Geometry check sheet. Reference: drawing and pictorial views, mm from the part's lowest x, y, z. Round coordinates to 2 decimals unless told otherwise and drop trailing zeros. Write each loop counter-clockwise with the first axis right and the second up, starting at its lowest first coordinate (ties: lowest second). Pieces come first, ordered by that corner, then holes. Notation, with made-up numbers: (-6, 25.25) - (22, 25.25) arc R34 cw to (22, 59.25) - close; hole circle Ø1 at (-17, 19). An arc over 180 degrees is marked (long way). Return JSON: item names as keys, results as strings.
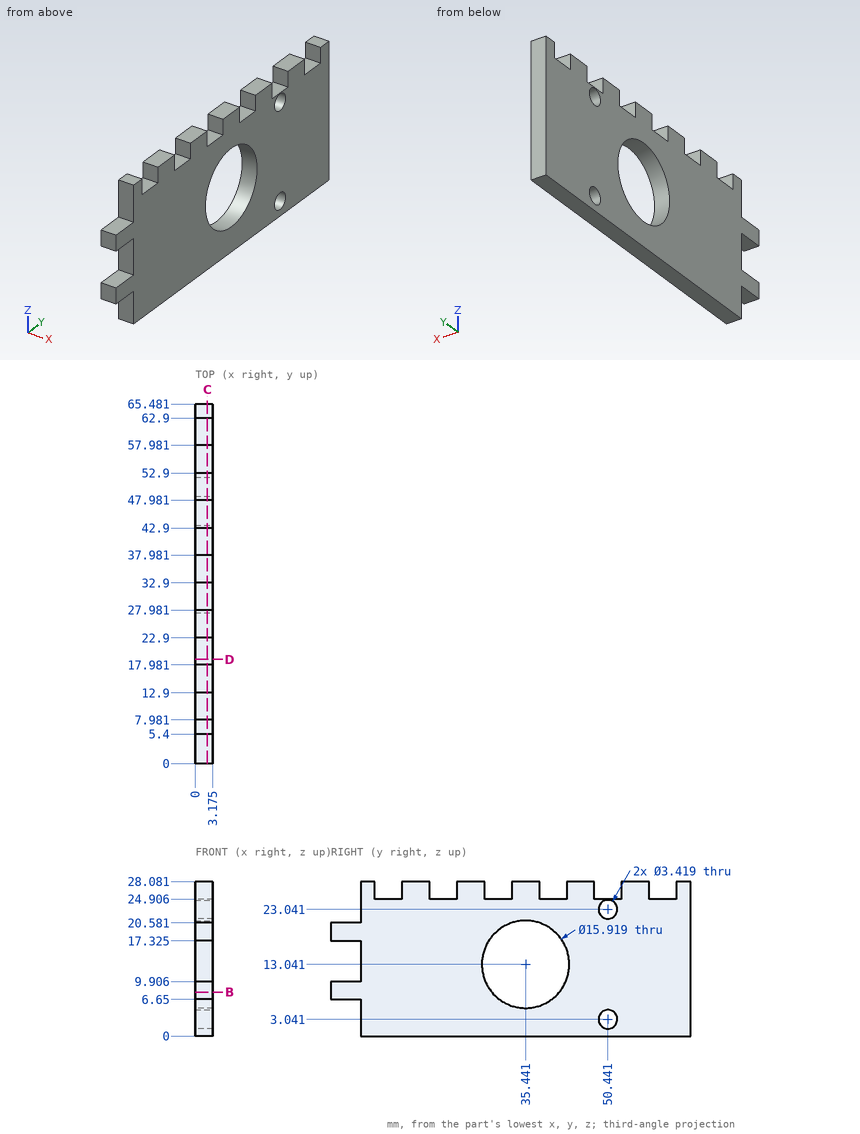
(1) Gauge pin test, flat ends, axial feed: pin 1 (1.6 mm diameter, centred on x = 1.5, z = 27, fed in from -Y); pin 2 (1.6 mm diameter, centred on x = 1, y = 11, fed in from +Z); pin 3 (2.5 mm diameter, centred on y = 50.44, z = 3.04, fed in from +X); pin 4 (3 mm diameter, centred on y = 56, z = 5, fed in from -X). Record the tip position at first contact, or that the pin passes through.
Response values:
{"pin 1": "stops at y = 5.4", "pin 2": "stops at z = 24.91", "pin 3": "passes through", "pin 4": "stops at x = 0"}
(2) Section check C-C, the plane x = 2.2. Give the number of separate pieces and of enclosed holes in the cut face, plus the area to 3 significant figures.
Response values:
{"separate pieces": "1", "enclosed holes": "3", "area": "1,410 mm^2"}
(3) Material ranges on line 1 along Z through (x, y) = (1.8, 50.5); line 2 along Z through (x, y) = (1.9, 50); line 3 along Z through (x, y) = (2, 12.5), recorded low to high. Write a range as [from, to].
Response values:
{"line 1": "z = [0, 1.33], [4.75, 21.33], [24.75, 24.91]", "line 2": "z = [0, 1.39], [4.69, 21.39], [24.69, 24.91]", "line 3": "z = [0, 24.91]"}
(4) Section check B-B, the plane z = 8. Enter the section's corners in (x, y) (1 decimal), plus the area to 3 significant figures.
Response values:
{"outline": "(0, 0) - (3.2, 0) - (3.2, 29.3) - (0, 29.3) - close; (0, 41.6) - (3.2, 41.6) - (3.2, 65.5) - (0, 65.5) - close", "area": "169 mm^2"}
(5) Section check D-D, the plane y = 19. Enter the section's corners in (x, z) (1 decimal).
Response values:
{"outline": "(0, 0) - (3.2, 0) - (3.2, 24.9) - (0, 24.9) - close"}
